For this review, take the finished solid that the model builds, in its own axes (mm). A direction names the side the tool comes from. Coordinates: 2 decimals unless noted, no trailing zeros. Loops run counter-clockwise (first coordinate to the right, second up) from the corner with the lowest first, then second, coordinate; pieces in that order, holes last.
1. Take a section at C-C, the plane y = -0.05. State the section outline as (x, z) points.
2. Mouldability with a two-part tool opening along Z and no side actions: class faces 1 (the face through (8, -24, 0)), 2 (the face through (2, 0, 24)), 3 (the face through (11.902, -22.028, -5.535)), 4 (the face through (2.46, -16.68, -14.42)) as pulls with the +Z half, pulls with the -Z half, needs draft (parallel to the pull), parting line crosses it, or undercut.
3. Machinability: for faces 5 (the face through (35, 20, 0)), 6 (the face through (9, -20, -4)), 7 (the face through (5, 0, 14)), 8 (the face through (19, -22, 0)), which of the approach directions +Z, -Z, +X, -X, +Y, -Y give a long, thin tool a straight path to every point of the face, cutting with its end or side? Answer none if there is none.
4. Take a section at B-B, the plane x = 31.6. State the section outline as (y, z) points.
5. Take a section at D-D, the plane z = -1.5. State the section outline as (x, y) points.
6. Take a section at A-A, the plane z = -15.5. State the section outline as (x, y) points.
7. To check wall thickness, follow probe 1 along Z at (x, y) = (3.6, -15.5); probe 2 along Y at (x, z) = (2, -15). State the ranges of each line that lie inside material, in increasing order.
8. Clearance check with flat-ended pins moving along their axes: P1, Ø4, axis at y = 15.5, z = 15.5, coming from the -X side; P2, Ø3.5, axis at y = -15.5, z = -15.5, coming from the +X side; P3, Ø1.2, axis at y = 21.5, z = -1, coming from the +X side; P4, Ø3, axis at x = 41.5, y = 11, coming from the -Z side. State where each tip first meets the part, or that it passes through.
```python
from build123d import *

# Parameters (mm, degrees)
SKETCH_W     = 48
SKETCH_H     = 48
SKETCH_R     = 1.6
PAD_DEPTH    = 5
SKETCH001_W  = 40
SKETCH001_H  = 6
PAD001_DEPTH = 52
PAD002_DEPTH = 4
PAD003_DEPTH = 4
SKETCH004_R  = 2.1
POCKET_DEPTH = 8
FILLET_R     = 6


with BuildPart() as part:
    # Sketch → Pad (new body)
    with BuildSketch(Plane.YZ):
        Rectangle(SKETCH_W, SKETCH_H)
        with Locations((-15.5, 15.5)):
            Circle(SKETCH_R, mode=Mode.SUBTRACT)
        with Locations((-15.5, -15.5)):
            Circle(SKETCH_R, mode=Mode.SUBTRACT)
        with Locations((15.5, -15.5)):
            Circle(SKETCH_R, mode=Mode.SUBTRACT)
        with Locations((15.5, 15.5)):
            Circle(SKETCH_R, mode=Mode.SUBTRACT)
    extrude(amount=PAD_DEPTH)

    # Sketch001 (on Face10 of Pad) → Pad001 (join)
    with BuildSketch(Plane.YZ.offset(5)):
        Rectangle(SKETCH001_W, SKETCH001_H)
    extrude(amount=PAD001_DEPTH)

    # Sketch002 (on DatumPlane) → Pad002 (join)
    with BuildSketch(Plane(origin=(0, -24, 0), x_dir=(0, 0, -1), z_dir=(0, -1, 0))):
        Polygon((-8, 5), (8, 5), (3, 19), (-3, 19), align=None)
    extrude(amount=-PAD002_DEPTH)

    # Sketch003 (on DatumPlane) → Pad003 (join)
    with BuildSketch(Plane.ZX.offset(24)):
        Polygon((-8, 5), (8, 5), (3, 19), (-3, 19), align=None)
    extrude(amount=-PAD003_DEPTH)

    # Sketch004 (on Face16 of Pad003) → Pocket (cut)
    with BuildSketch(Plane(origin=(0, 0, 3), x_dir=(0, -1, 0), z_dir=(0, 0, 1))):
        with Locations((0.05, 50.65)):
            Circle(SKETCH004_R)
        with Locations((12.75, 31.6)):
            Circle(SKETCH004_R)
    extrude(amount=-POCKET_DEPTH, mode=Mode.SUBTRACT)

    # Fillet
    fillet_edges = [part.edges().sort_by_distance(p)[0] for p in [
        (2.5, -24, 24),
        (57, -20, 0),
        (57, 20, 0),
        (2.5, -24, -24),
        (2.5, 24, -24),
        (2.5, 24, 24),
    ]]
    fillet(fillet_edges, radius=FILLET_R)


solid = part.part
```
Results list:
1. outline: (0, -24) - (5, -24) - (5, -3) - (48.55, -3) - (48.55, 3) - (5, 3) - (5, 24) - (0, 24) - close; (52.75, -3) - (57, -3) - (57, 3) - (52.75, 3) - close
2. face 1: needs draft
2. face 2: pulls with the +Z half
2. face 3: pulls with the -Z half
2. face 4: undercut
3. face 5: +Z, -Z, +X, +Y
3. face 6: -Z, +X
3. face 7: +Z, +X
3. face 8: +Z, -Z, +X, -Y
4. outline: (-20, -3) - (-14.85, -3) - (-14.85, 3) - (-20, 3) - close; (-10.65, -3) - (20, -3) - (20, 3) - (-10.65, 3) - close
5. outline: (0, -24) - (19, -24) - (19, -20) - (51, -20) arc R6 ccw to (57, -14) - (57, 14) arc R6 ccw to (51, 20) - (19, 20) - (19, 24) - (0, 24) - close; hole circle Ø4.2 at (31.6, -12.75); hole circle Ø4.2 at (50.65, -0.05)
6. outline: (0, -24) - (5, -24) - (5, -17.1) - (0, -17.1) - close; (0, -13.9) - (5, -13.9) - (5, 13.9) - (0, 13.9) - close; (0, 17.1) - (5, 17.1) - (5, 24) - (0, 24) - close
7. probe 1: z = -24 to -17.1, -13.9 to 13.9, 17.1 to 24
7. probe 2: y = -24 to -17.02, -13.98 to 13.98, 17.02 to 24
8. P1: stops at x = 0
8. P2: stops at x = 5
8. P3: stops at x = 19
8. P4: stops at z = -3
